Answer from the drawing. Dimensions are ordinates in mm from the lowest x, y and z of the part. Coordinates: 2 decimals unless noted, no trailing zeros. Order: outer loops, then holes, each group sorted by start corner. A loop starts at its lowest first (then second) coordinate and runs counter-clockwise, first axis right, second up. Notation, with made-up numbers: (-0.5, 0.25) -> (44.5, 0.25) arc R16 ccw to (44.5, 15.25) -> close; hole circle Ø4 at (85, 72.5). An arc over 180 degrees is marked (long way). Use CSV: the item, a comma, the result in double quotes.
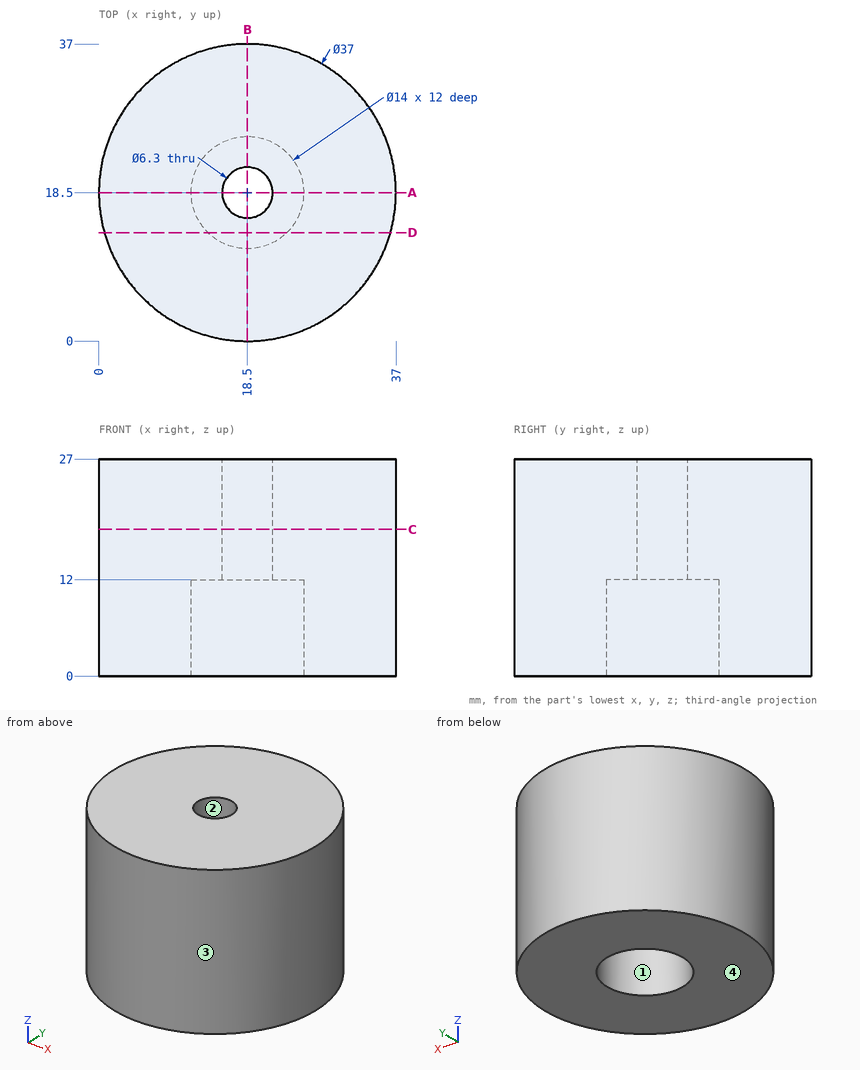
Item 1: Each of these flat-tipped pins is pushed along its axis until it touches: P1, Ø5, axis at y = 26, z = 6, coming from the -X side; P2, Ø8, axis at x = 15.5, z = 3.5, coming from the -Y side; P3, Ø2, axis at x = 17.5, z = 16.5, coming from the +Y side. Where does it stop, or does it pass through?
Return value:
P1,"stops at x = 0.69"
P2,"stops at y = 0"
P3,"stops at y = 37"
Item 2: Find section A-A, the plane y = 18.5. Give the vertices of the cut face in (x, z).
Return value:
outline,"(0, 0) -> (11.5, 0) -> (11.5, 12) -> (15.35, 12) -> (15.35, 27) -> (0, 27) -> close; (21.65, 12) -> (25.5, 12) -> (25.5, 0) -> (37, 0) -> (37, 27) -> (21.65, 27) -> close"
Item 3: The mould has two halves that part along X. Classify the marked faces 1, 2, 3 and 4: +X half, -X half, draft (parallel to the pull), parting line (faces both ways), or undercut.
Return value:
face 1,"undercut"
face 2,"undercut"
face 3,"parting line"
face 4,"draft"
Item 4: Find section D-D, the plane y = 13.5. Give the vertices of the cut face in (x, z), then the cut area to 3 significant figures.
Return value:
outline,"(0.69, 0) -> (13.6, 0) -> (13.6, 12) -> (23.4, 12) -> (23.4, 0) -> (36.31, 0) -> (36.31, 27) -> (0.69, 27) -> close"
area,"844 mm^2"
Item 5: Straight lines are drawn through the part: line 1 along Y through (x, z) = (18.5, 18.75); line 2 along Z through (x, y) = (22, 19); line 3 along Y through (x, z) = (18.5, 8.5). For each, find the intervals that lie inside material, in ascending order.
Return value:
line 1,"y = 0 to 15.35, 21.65 to 37"
line 2,"z = 12 to 27"
line 3,"y = 0 to 11.5, 25.5 to 37"
Item 6: Find section C-C, the plane z = 18.25. Give the vertices of the cut face in (x, y), then the cut area to 3 significant figures.
Return value:
outline,"circle Ø37 at (18.5, 18.5); hole circle Ø6.3 at (18.5, 18.5)"
area,"1,040 mm^2"
